```python
from build123d import *

# Parameters (mm, degrees)
F0_R     = 6.5
F1_DEPTH = 13
F2_R     = 3
F3_DEPTH = 35
F4_SIZE2 = 0.528981
F4_SIZE  = 3
F5_SIZE  = 1


with BuildPart() as f1:
    # F0 (on Front) → F1 (new body)
    with BuildSketch(Plane.XZ):
        Circle(F0_R)
    extrude(amount=-F1_DEPTH)

    # F2 (on face) → F3 (join)
    with BuildSketch(Plane(origin=(0, 13, 0), x_dir=(-1, 0, 0), z_dir=(0, 1, 0))):
        Circle(F2_R)
    extrude(amount=F3_DEPTH)

    # F4
    f4_edges = [f1.edges().sort_by_distance(p)[0] for p in [
        (3, 48, 0),
    ]]
    chamfer(f4_edges, length=F4_SIZE, length2=F4_SIZE2)

    # F5
    f5_edges = [f1.edges().sort_by_distance(p)[0] for p in [
        (-6.5, 13, 0),
        (-6.5, 0, 0),
    ]]
    chamfer(f5_edges, length=F5_SIZE)

    # F6 (on Right) → F7 (revolve, cut)
    with BuildSketch(Plane.YZ):
        with BuildLine():
            Line((12, 7.074941), (1, 7.082712))
            ThreePointArc((1, 7.082712), (6.498825, 5.41508), (12, 7.074941))
        make_face()
    revolve(axis=Axis((0, 13, 0), (0, -1, 0)), mode=Mode.SUBTRACT)


solid = f1.part
```
For this review, take the finished solid that the model builds, in its own axes (mm). A direction names the side the tool comes from. Round coordinates to 2 decimals unless told otherwise and drop trailing zeros. Write each loop counter-clockwise with the first axis right and the second up, starting at its lowest first coordinate (ties: lowest second). Pieces come first, ordered by that corner, then holes. Notation, with made-up numbers: (49, 42.5) -> (80, 42.5) arc R19 ccw to (80, 70.5) -> close; hole circle Ø3 at (-20.5, 30.5). An arc over 180 degrees is marked (long way). One line per question, with ' | ' between items. Start each with the question number.
1) Add section C-C (y = 26). Write out the cut boundary in (x, z).
2) Machinability: for faces 1 (the flat face through (2.4, 13, -2.4)), 2 (the cylindrical face through (-5.158, 1.49, -3.955)), which of the approach directions +Z, -Z, +X, -X, +Y, -Y give a long, thin tool a straight path to every point of the face, cutting with its end or side? Answer none if there is none.
3) Add section B-B (x = 0). Write out the cut boundary in (y, z).
4) Wall thickness on line 1 along Z through (x, y) = (0.25, 45); line 2 along Y through (x, z) = (2.25, 5.75); line 3 along Y through (x, z) = (2.25, 4.25): over which ranges is each line inside the solid? List them lowest first.
5) For pin 1 Ø2 at (x, z) = (-2.5, -1) entering from -Y; pin 2 Ø6 at (y, z) = (18.5, 0) entering from +X, all flat-tipped, find the tip position at first contact; note any pin that passes through.
6) Add section A-A (z = 0). Write out the cut boundary in (x, y), and give its area (3 significant figures).
Reported:
1) outline: circle Ø6 at (0, 0)
2) face 1: +Y | face 2: +Y, -Y
3) outline: (0, -5.5) -> (1, -6.5) -> (1.99, -6.5) arc R9.92 cw to (11.02, -6.5) -> (12, -6.5) -> (13, -5.5) -> (13, -3) -> (45, -3) -> (48, -2.47) -> (48, 2.47) -> (45, 3) -> (13, 3) -> (13, 5.5) -> (12, 6.5) -> (11.02, 6.5) arc R9.92 cw to (1.99, 6.5) -> (1, 6.5) -> (0, 5.5) -> close
4) line 1: z = -2.99 to 2.99 | line 2: y = 0.67 to 2.7, 10.31 to 12.33 | line 3: y = 0 to 13
5) pin 1: stops at y = 0 | pin 2: stops at x = 3
6) outline: (-6.5, 1) -> (-5.5, 0) -> (5.5, 0) -> (6.5, 1) -> (6.5, 1.99) arc R9.92 cw to (6.5, 11.02) -> (6.5, 12) -> (5.5, 13) -> (3, 13) -> (3, 45) -> (2.47, 48) -> (-2.47, 48) -> (-3, 45) -> (-3, 13) -> (-5.5, 13) -> (-6.5, 12) -> (-6.5, 11.02) arc R9.92 cw to (-6.5, 1.99) -> close | area: 362 mm²
